Could you check a few things on this model? Use its own coordinates, in mm. Face numbers are marked on the shaded views. A direction names the side the tool comes from. Give positions to 0.01 mm unless a question says otherwise; leave off trailing zeros. Write each loop counter-clockwise with the first axis right and the second up, starting at its lowest first coordinate (ties: lowest second). Pieces come first, ordered by that corner, then holes. Notation, with made-up numbers: (-5.75, 79.5) - (42.25, 79.5) arc R19 ccw to (42.25, 87.5) - close; hole circle Ø1 at (-20, 89.25). An arc over 180 degrees is marked (long way). Answer as CSV lines item,"result". Start each with the question number.
Q1. On a 3-axis mill with a long thin cutter (end or side, diameter ignored), from which of +Z, -Z, +X, -X, +Y, -Y can I reach the whole of each face in a straight line? I mean the marked faces 1, 2 and 3. Say none if no direction works.
Q2. Imagine slicing it at B-B on x = -43.5. List the corners of the cut face in (y, z) for me.
Q3. Will these pins go through, and if not, where does the flat tip stop? pin 1 Ø1.3 at (x, z) = (-1.5, -5.5) entering from -Y; pin 2 Ø4 at (x, z) = (28, 2.5) entering from -Y; pin 3 Ø2 at (x, y) = (-22.5, 0) entering from -Z.
Q4. Imagine slicing it at A-A on z = 4. List the corners of the cut face in (x, y) for me, and give its area (3 significant figures).
Q5. If I drill on line 1 along Y through (x, z) = (-43.5, 2.9); line 2 along Z through (x, y) = (10, -1); line 3 along X through (y, z) = (-12, -5), over which ranges is the centre line in solid material (lowest first)?
Q6. Imagine slicing it at D-D on x = -12. List the corners of the cut face in (y, z) for me, and give its area (3 significant figures).
Q7. Imagine slicing it at C-C on y = 0. List the corners of the cut face in (x, z) for me.
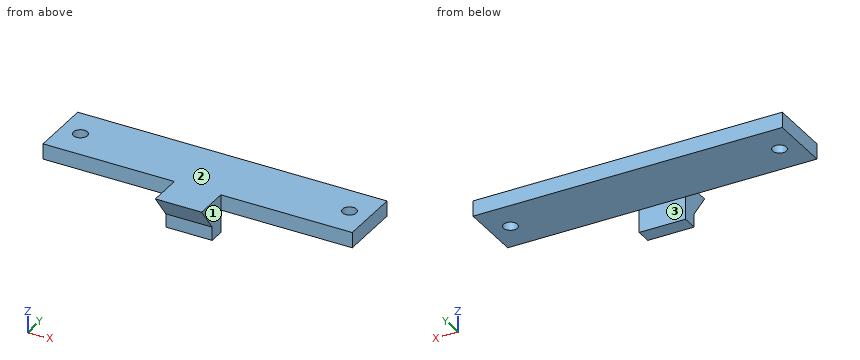
```python
from build123d import *

# Parameters (mm, degrees)
SKETCH_1_W          = 100
SKETCH_1_H          = 20
EXTRUDE_1_DEPTH     = 5
HOLE_WIZARD_M4_1_D  = 4.5
SKETCH_4_W          = 15
SKETCH_4_H          = 5
EXTRUDE_2_DEPTH     = 5
SKETCH_5_W          = 15
SKETCH_5_H          = 5
EXTRUDE_3_DEPTH     = 7.35
SKETCH_6_W          = 15
SKETCH_6_H          = 8
EXTRUDE_4_DEPTH     = 6
CUT_EXTRUDE_1_DEPTH = 62.654460504


with BuildPart() as part:
    # 스케치1 → 보스-돌출1 (new body)
    with BuildSketch(Plane.XY):
        Rectangle(SKETCH_1_W, SKETCH_1_H)
    extrude(amount=EXTRUDE_1_DEPTH)

    # M4 여유 구멍1 (through all)
    with Locations(Plane.XY.offset(5)):
        with Locations((-43.5, 0), (43.5, 0)):
            Hole(HOLE_WIZARD_M4_1_D / 2)

    # 스케치4 → 보스-돌출2 (add)
    with BuildSketch(Plane(origin=(0, -10, 0), x_dir=(1, 0, 0), z_dir=(0, 1, 0))):
        with Locations((0, -2.5)):
            Rectangle(SKETCH_4_W, SKETCH_4_H)
    extrude(amount=-EXTRUDE_2_DEPTH)

    # 스케치5 → 보스-돌출3 (add)
    with BuildSketch(Plane.XY):
        with Locations((0, -12.5)):
            Rectangle(SKETCH_5_W, SKETCH_5_H)
    extrude(amount=-EXTRUDE_3_DEPTH)

    # 스케치6 → 보스-돌출4 (add)
    with BuildSketch(Plane.XZ.offset(15)):
        with Locations((0, 1)):
            Rectangle(SKETCH_6_W, SKETCH_6_H)
    extrude(amount=EXTRUDE_4_DEPTH)

    # 스케치7 → 컷-돌출1 (cut, through all)
    with BuildSketch(Plane(origin=(7.5, 0, 0), x_dir=(0, 0, -1), z_dir=(1, 0, 0))):
        Polygon((3, -21), (-5, -21), (3, -15), align=None)
    extrude(amount=-CUT_EXTRUDE_1_DEPTH, mode=Mode.SUBTRACT)


solid = part.part
```
Conclusion:
1,face 1,"+Z, -Z, +X, -Y"
1,face 2,"+Z, +X, -X, +Y, -Y"
1,face 3,"-Z, +X, -X, +Y"
2,outline,"(-10, 0) - (-2.25, 0) - (-2.25, 5) - (-10, 5) - close; (2.25, 0) - (10, 0) - (10, 5) - (2.25, 5) - close"
3,pin 1,"y = -15"
3,pin 2,"y = -10"
3,pin 3,"z = 0"
4,outline,"(-50, -10) - (-7.5, -10) - (-7.5, -20.25) - (7.5, -20.25) - (7.5, -10) - (50, -10) - (50, 10) - (-50, 10) - close; hole circle Ø4.5 at (-43.5, 0); hole circle Ø4.5 at (43.5, 0)"
4,area,"2,120 mm^2"
5,line 1,"-10 to -2.25, 2.25 to 10"
5,line 2,"0 to 5"
5,line 3,"-7.5 to 7.5"
6,outline,"(-10, 0) - (10, 0) - (10, 5) - (-10, 5) - close"
6,area,"100 mm^2"
7,outline,"(-50, 0) - (-45.75, 0) - (-45.75, 5) - (-50, 5) - close; (-41.25, 0) - (41.25, 0) - (41.25, 5) - (-41.25, 5) - close; (45.75, 0) - (50, 0) - (50, 5) - (45.75, 5) - close"
